Autodesk Inventor part; units mm, degrees
ref_plane "YZ Plane" through (0, 0, 0) normal (1, 0, 0) x (0, 1, 0)
ref_plane "XZ Plane" through (0, 0, 0) normal (0, 1, 0) x (-1, 0, 0)
ref_plane "XY Plane" through (0, 0, 0) normal (0, 0, 1) x (1, 0, 0)
sketch "Sketch2" plane through (0, 0, 0) normal (0, 1, 0) x (-1, 0, 0)
  line L0 (90, -53) -> (84, -53)
  line L1 (84, -53) -> (84, -43)
  line L2 (84, -43) -> (90, -43)
  line L3 (-90, -53) -> (-84, -53)
  line L4 (-84, -53) -> (-84, -43)
  line L5 (-84, -43) -> (-90, -43)
  line L6 (70, -18) -> (60, -18)
  line L7 (60, -18) -> (60, -15)
  line L8 (60, -15) -> (70, -15)
  line L9 (70, -15) -> (70, -18)
  line L10 (-70, -18) -> (-60, -18)
  line L11 (-60, -18) -> (-60, -15)
  line L12 (-60, -15) -> (-70, -15)
  line L13 (-70, -15) -> (-70, -18)
  circle A0 centre (0, 0) radius 41.275
  line L14 (46.5, -15) -> (43.5, -15)
  line L15 (43.5, -15) -> (43.5, -5)
  line L16 (43.5, -5) -> (46.5, -5)
  line L17 (46.5, -5) -> (46.5, -15)
  line L18 (-46.5, -15) -> (-43.5, -15)
  line L19 (-43.5, -15) -> (-43.5, -5)
  line L20 (-43.5, -5) -> (-46.5, -5)
  line L21 (-46.5, -5) -> (-46.5, -15)
  line L22 (43.5, 57) -> (43.5, 47)
  line L23 (43.5, 47) -> (46.5, 47)
  line L24 (46.5, 47) -> (46.5, 57)
  line L25 (-46.5, 47) -> (-43.5, 47)
  line L26 (-43.5, 47) -> (-43.5, 57)
  line L27 (-46.5, 57) -> (-46.5, 47)
  line L28 (-22.7645, 85) -> (22.7645, 85)
  line L29 (46.5, 57) -> (43.5, 57)
  line L30 (-43.5, 57) -> (-46.5, 57)
  line L31 (30, 57) -> (20, 57)
  line L32 (20, 57) -> (20, 60)
  line L33 (20, 60) -> (30, 60)
  line L34 (30, 60) -> (30, 57)
  line L35 (-20, 57) -> (-30, 57)
  line L36 (-30, 57) -> (-30, 60)
  line L37 (-30, 60) -> (-20, 60)
  line L38 (-20, 60) -> (-20, 57)
  line L39 (4.5, 70) -> (-4.5, 70)
  line L40 (-4.5, 70) -> (-4.5, 80)
  line L41 (-4.5, 80) -> (4.5, 80)
  line L42 (4.5, 80) -> (4.5, 70)
  line L43 (4.5, 45) -> (-4.5, 45)
  line L44 (-4.5, 45) -> (-4.5, 55)
  line L45 (-4.5, 55) -> (4.5, 55)
  line L46 (4.5, 55) -> (4.5, 45)
  line L47 (-90, -43) -> (-90, -7.5731)
  line L48 (90, -7.5731) -> (90, -43)
  line L49 (90, -53) -> (90, -65)
  line L50 (-90, -53) -> (-90, -65)
  line L51 (90, -65) -> (-90, -65)
  line L52 (-62, 17.5731) -> (-62, 61.9813)
  line L53 (-59.3287, 66.4059) -> (-25.0933, 84.4246)
  line L54 (-64.0938, 13.5044) -> (-87.9062, -3.5044)
  line L55 (87.9062, -3.5044) -> (64.0938, 13.5044)
  line L56 (62, 17.5731) -> (62, 61.9813)
  line L57 (59.3287, 66.4059) -> (25.0933, 84.4246)
  arc A1 (-87.9062, -3.5044) -> (-90, -7.5731) centre (-85, -7.5731) ccw
  arc A2 (-64.0938, 13.5044) -> (-62, 17.5731) centre (-67, 17.5731) ccw
  arc A3 (-59.3287, 66.4059) -> (-62, 61.9813) centre (-57, 61.9813) ccw
  arc A4 (-22.7645, 85) -> (-25.0933, 84.4246) centre (-22.7645, 80) ccw
  arc A5 (25.0933, 84.4246) -> (22.7645, 85) centre (22.7645, 80) ccw
  arc A6 (62, 61.9813) -> (59.3287, 66.4059) centre (57, 61.9813) ccw
  arc A7 (62, 17.5731) -> (64.0938, 13.5044) centre (67, 17.5731) ccw
  arc A8 (90, -7.5731) -> (87.9062, -3.5044) centre (85, -7.5731) ccw
  point P0 (-62, 15)
  point P1 (-62, 65)
  point P2 (0, 0)
  point P3 (-24, 85)
  point P4 (-90, -5)
  point P5 (62, 15)
  point P6 (62, 65)
  point P7 (90, -5)
  point P8 (24, 85)
  dimension "d21" = 6
  dimension "d22" = 10
  dimension "d25" = 6
  dimension "d26" = 10
  dimension "d31" = 3
  dimension "d32" = 10
  dimension "d35" = 3
  dimension "d36" = 10
  dimension "d39" = 25
  dimension "d40" = 25
  dimension "d43" = 82.55
  dimension "d52" = 3
  dimension "d53" = 10
  dimension "d54" = 10
  dimension "d55" = 3
  dimension "d58" = 10
  dimension "d59" = 3
  dimension "d62" = 3
  dimension "d65" = 180
  dimension "d90" = 90
  dimension "d91" = 90
  dimension "d103" = 10
  dimension "d104" = 10
  dimension "d108" = 3
  dimension "d109" = 10
  dimension "d110" = 20
  dimension "d111" = 3
  dimension "d112" = 10
  dimension "d113" = 20
  dimension "d114" = 5
  dimension "d115" = 10
  dimension "d116" = 9
  dimension "d117" = 4.5
  dimension "d118" = 10
  dimension "d119" = 9
  dimension "d120" = 15
  dimension "d121" = 4.5
  dimension "d127" = 180
  dimension "d128" = 150
  dimension "d130" = 85.5
  dimension "d131" = 43.5
  dimension "d132" = 43.5
  dimension "d133" = 60
  dimension "d134" = 60
  dimension "d135" = 43.5
  dimension "d136" = 43.5
  dimension "d137" = 90
  dimension "d138" = 28
  dimension "d140" = 47
  dimension "d141" = 47
  dimension "d144" = 60
  dimension "d145" = 20
  dimension "d147" = 65
  dimension "d149" = 50
  dimension "d151" = 10
  dimension "d152" = 60
  dimension "d153" = 20
  dimension "d154" = 50
  dimension "d155" = 62
  dimension "d156" = 62
  dimension "d157" = 62
  dimension "d158" = 57
  dimension "d159" = 57
  dimension "d160" = 3
extrude "Extrusion6" add sketch "Sketch2" along normal blind 3
properties part number "Top Plate 25090213"
Source: CAD feature listing. Evaluate the final solid. Frame: model axes, mm. Round coordinates to 2 decimals unless told otherwise and drop trailing zeros. Loops run counter-clockwise (first coordinate to the right, second up) from the corner with the lowest first, then second, coordinate; pieces in that order, holes last. Notation, with made-up numbers: (80, 70.25) - (115, 70.25) arc R20 ccw to (115, 95.25) - close; hole circle Ø11 at (20, 31.25). An arc over 180 degrees is marked (long way). Write item = value, one per line. Start each with the question number.
(1) Ray query, line 1 along Z through (x, y) = (0, 1.5) (3 decimals); line 2 along X through (y, z) = (0.55, 54.5); line 3 along X through (y, z) = (1.3, 59.5). Return the intervals inside material, ascending. Write a range as from..to.
(2) Pin query (flat end, axial travel): pin 1 (1 mm diameter, centred on x = -71, y = 1.5, fed in from +Z); pin 2 (1.5 mm diameter, centred on x = -44.5, y = 2, fed in from +Z); pin 3 (0.9 mm diameter, centred on x = -25.5, y = 2, fed in from +Z). Return the tip coordinate at first contact, or that it passes through.
(3) Pull-direction query (Z, two-part tool) for faces 1 (the face through (41, 3, -6)), 2 (the face through (8.948, 1.479, 40.293)), 3 (the face through (42.45, 1.48, 75.29)); classes: +Z half, -Z half, draft (parallel to the pull), parting line (faces both ways), or undercut.
(4) Section query D-D, the plane z = 29. Output: boundary loops of the cut face in (x, y), plus the area to 3 significant figures.
(5) Section query C-C, the plane y = 1.5. State how many separate pieces and enclosed holes the cut face has, plus the area to 3 significant figures.
(6) Section query B-B, the plane z = 0. Output: boundary loops of the cut face in (x, y) (3 decimals).
(7) Section query A-A, the plane x = 0. Output: boundary loops of the cut face in (y, z) (3 decimals).
Conclusion:
q1.line_1 = -65..-41.275, 41.275..45, 55..70, 80..85
q1.line_2 = -62..-46.5, -43.5..-4.5, 4.5..43.5, 46.5..62
q1.line_3 = -62..-30, -20..20, 30..62
q2.pin_1 = 8.93
q2.pin_2 = 74.61
q2.pin_3 = 84.45
q3.face_1 = draft
q3.face_2 = undercut
q3.face_3 = +Z half
q4.outline = (-62, 0) - (-29.37, 0) - (-29.37, 3) - (-62, 3) - close; (29.37, 0) - (62, 0) - (62, 3) - (29.37, 3) - close
q4.area = 196 mm2
q5.separate_pieces = 1
q5.enclosed_holes = 11
q5.area = 15,900 mm2
q6.outline = (-83, 0) - (-41.275, 0) - (-41.275, 3) - (-83, 3) - close; (41.275, 0) - (83, 0) - (83, 3) - (41.275, 3) - close
q7.outline = (0, -65) - (3, -65) - (3, -41.275) - (0, -41.275) - close; (0, 41.275) - (3, 41.275) - (3, 45) - (0, 45) - close; (0, 55) - (3, 55) - (3, 70) - (0, 70) - close; (0, 80) - (3, 80) - (3, 85) - (0, 85) - close
